Build history of the part. All positions in model axes, mm. Face numbers are marked on the shaded views. A direction names the side the tool comes from. Round coordinates to 2 decimals unless told otherwise and drop trailing zeros. Write each loop counter-clockwise with the first axis right and the second up, starting at its lowest first coordinate (ties: lowest second). Pieces come first, ordered by that corner, then holes. Notation, with made-up numbers: M -29,89.25 L 3,89.25 A18 cw 3,115.25 Z; hole C -6,-7 d9. An arc over 180 degrees is marked long. Use a Markdown table: item, result.
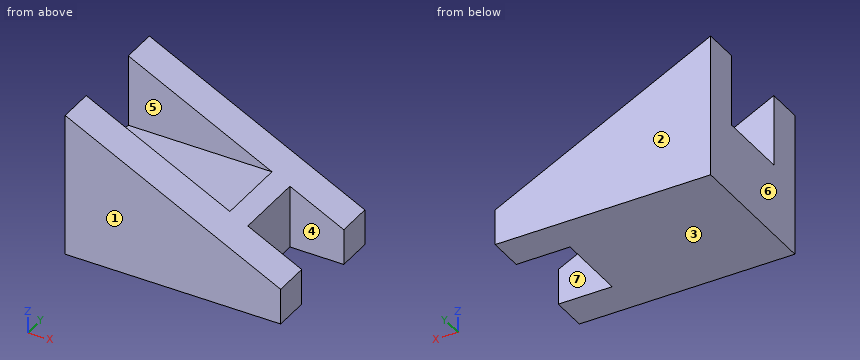
from build123d import *

# Parameters (mm, degrees)
F1_DEPTH = 20
F2_W     = 10
F2_H     = 10
F3_DEPTH = 25
F4_W     = 7.5
F4_H     = 10
F5_DEPTH = 25


with BuildPart() as f1:
    # F0 (on Front) → F1 (new body)
    with BuildSketch(Plane.XZ):
        Polygon((0, 20), (0, 0), (30, 0), (30, 5), align=None)
    extrude(amount=-F1_DEPTH)

    # F2 (on Right) → F3 (cut)
    with BuildSketch(Plane.YZ):
        with Locations((10, 15)):
            Rectangle(F2_W, F2_H)
    extrude(amount=F3_DEPTH, mode=Mode.SUBTRACT)

    # F4 (on Top) → F5 (cut)
    with BuildSketch(Plane.XY):
        with Locations((26.25, 10)):
            Rectangle(F4_W, F4_H)
    extrude(amount=F5_DEPTH, mode=Mode.SUBTRACT)


solid = f1.part
Q1. Drill centre lines: L1, parallel to Y at x = 1.5, z = 13.75; L2, parallel to X at y = 11.25, z = 7.5; L3, parallel to Z at x = 6, y = 13.5. Where is each one in solid material? Low to high.
Response values:
| item | result |
|---|---|
| L1 | y = 0 to 5, 15 to 20 |
| L2 | x = 0 to 22.5 |
| L3 | z = 0 to 10 |
Q2. Cut at B-B on x = 23. Give the cut face in (y, z), and give its area (3 significant figures).
Response values:
| item | result |
|---|---|
| outline | M 0,0 L 5,0 L 5,8.5 L 0,8.5 Z; M 15,0 L 20,0 L 20,8.5 L 15,8.5 Z |
| area | 85.0 mm2 |
Q3. Which spindle directions (+Z, -Z, +X, -X, +Y, -Y) get a long thin tool onto all of the face, cutting with end or side? Do the marked faces 5, 6 and 7. Say none if no direction does.
Response values:
| item | result |
|---|---|
| face 5 | +Z, +X, -X |
| face 6 | +Z, -Z, -X, +Y, -Y |
| face 7 | +Z, -Z, +X |
Q4. Cut at A-A on z = 11.75. Give the cut face in (x, y), and give its area (3 significant figures).
Response values:
| item | result |
|---|---|
| outline | M 0,0 L 16.5,0 L 16.5,5 L 0,5 Z; M 0,15 L 16.5,15 L 16.5,20 L 0,20 Z |
| area | 165 mm2 |
Q5. Cut at D-D on y = 17.25. Give the cut face in (x, z), and give its area (3 significant figures).
Response values:
| item | result |
|---|---|
| outline | M 0,0 L 30,0 L 30,5 L 0,20 Z |
| area | 375 mm2 |
Q6. Two-plate mould, pull along Y, no slides. Class the marked faces 1, 2, 3 and 4: +Y half, -Y half, draft (parallel to the pull), parting line (faces both ways), or undercut.
Response values:
| item | result |
|---|---|
| face 1 | -Y half |
| face 2 | +Y half |
| face 3 | draft |
| face 4 | undercut |
Q7. Cut at C-C on x = 16. Give the cut face in (y, z).
Response values:
| item | result |
|---|---|
| outline | M 0,0 L 20,0 L 20,12 L 15,12 L 15,10 L 5,10 L 5,12 L 0,12 Z |
Q8. Drop flat-ended pins along their axis: P1, Ø5, axis at x = 15.5, y = 13, coming from the +Z side; P2, Ø8, axis at x = 26, z = 4.5, coming from the -Y side; P3, Ø4, axis at x = 10, y = 7.5, coming from the +Z side; P4, Ø8, axis at x = 11, y = 12, coming from the +Z side. Give the stop position or say it passes through.
Response values:
| item | result |
|---|---|
| P1 | stops at z = 13 |
| P2 | stops at y = 0 |
| P3 | stops at z = 10 |
| P4 | stops at z = 15.82 |
